Geometry check sheet. Reference: the model listing, model coordinates, mm. Round coordinates to 2 decimals unless told otherwise and drop trailing zeros. Order: outer loops, then holes, each group sorted by start corner. A loop starts at its lowest first (then second) coordinate and runs counter-clockwise, first axis right, second up.
```python
from build123d import *

# Parameters (mm, degrees)
F0_R     = 9.75
F0_R_2   = 7.75
F1_DEPTH = 5
F2_R     = 1.99999
F3_R     = 1.99999


# Not quite as in the source:
# - a fillet or chamfer is up to 0.001 mm smaller than in the source, because OpenCascade refuses the exact size


with BuildPart() as f1:
    # F0 (on Right) → F1 (new body)
    with BuildSketch(Plane.YZ):
        Circle(F0_R)
        Circle(F0_R_2, mode=Mode.SUBTRACT)
    extrude(amount=F1_DEPTH)

    # F2 (radius 2 in the source; OpenCascade refuses exactly that, so slightly less here)
    f2_edges = [f1.edges().sort_by_distance(p)[0] for p in [
        (0, -9.75, 0),
    ]]
    fillet(f2_edges, radius=F2_R)

    # F3 (radius 2 in the source; OpenCascade refuses exactly that, so slightly less here)
    f3_edges = [f1.edges().sort_by_distance(p)[0] for p in [
        (5, -9.75, 0),
    ]]
    fillet(f3_edges, radius=F3_R)


solid = f1.part
```
(1) Draft check along Y on faces 1 (the cylindrical face through (2.493, -1.269, 9.667)), 2 (the cylindrical face through (2.465, -1.009, 7.684)). Enter one of: released by +Y, released by -Y, zero draft, split by the parting line, or undercut.
Returned:
face 1: split by the parting line
face 2: undercut
(2) Sectioned sample at C-C, the plane x = 4.75. Record the cut outline in (y, z).
Returned:
outline: circle Ø17.44 at (0, 0); hole circle Ø15.5 at (0, 0)
(3) Depth check by flat-ended pin: P1, Ø1, axis at x = 2, y = 7, coming from the +Z side. Enter the tip coordinate at first touch or a pass-through.
Returned:
P1: stops at z = 7.27
(4) Material ranges on line 1 (Z direction, x = 2.7, y = -4.5); line 2 (Z direction, x = 1.7, y = 0); line 3 (Y direction, x = 0.7, z = -3.5), recorded low to high.
Returned:
line 1: z = -8.65 to -6.31, 6.31 to 8.65
line 2: z = -9.73 to -7.75, 7.75 to 9.73
line 3: y = -8.58 to -6.91, 6.91 to 8.58
(5) Sectioned sample at D-D, the plane x = 0.9. Record the cut outline in (y, z).
Returned:
outline: circle Ø18.84 at (0, 0); hole circle Ø15.5 at (0, 0)
